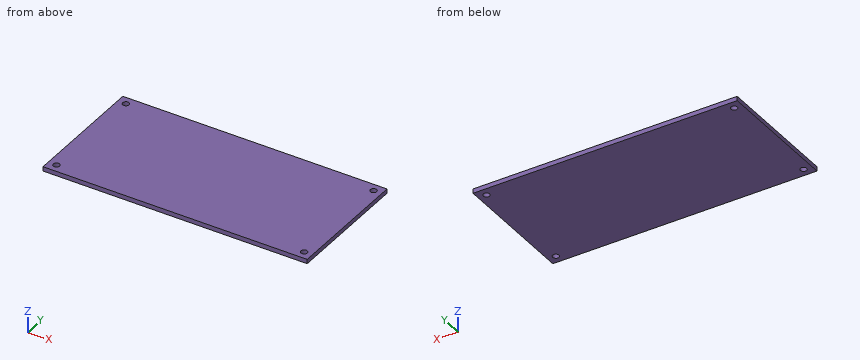
from build123d import *

# Parameters (mm, degrees)
ESQUISSE1_W        = 96
ESQUISSE1_H        = 46
ESQUISSE1_R        = 1.15
BOSS_EXTRU_1_DEPTH = 1.6


with BuildPart() as part:
    # Esquisse1 → Boss.-Extru.1 (new body)
    with BuildSketch(Plane.XY):
        Rectangle(ESQUISSE1_W, ESQUISSE1_H)
        with Locations((-45, 20)):
            Circle(ESQUISSE1_R, mode=Mode.SUBTRACT)
        with Locations(Location((45, 20, 0), (0, 0, 180))):
            Circle(ESQUISSE1_R, mode=Mode.SUBTRACT)
        with Locations(Location((-45, -20, 0), (0, 0, 180))):
            Circle(ESQUISSE1_R, mode=Mode.SUBTRACT)
        with Locations((45, -20)):
            Circle(ESQUISSE1_R, mode=Mode.SUBTRACT)
    extrude(amount=BOSS_EXTRU_1_DEPTH)


solid = part.part
Work out the finished part from the listing and answer in its coordinate system (mm). Give positions to 0.01 mm unless a question says otherwise; leave off trailing zeros. Write each loop counter-clockwise with the first axis right and the second up, starting at its lowest first coordinate (ties: lowest second). Pieces come first, ordered by that corner, then holes. Notation, with made-up numbers: (-9.5, 4) - (-4.5, 4) arc R27 ccw to (-4.5, 21) - close; hole circle Ø4 at (-36, -1.5). An arc over 180 degrees is marked (long way). One line per item, written item: value. Start each with the question number.
1. Given pin 1 (10 mm diameter, centred on x = -15.5, y = 3.5, fed in from -Z), flat-ended and moving along its own axis, determine where the tip first touches the part or whether it passes through.
2. Find section B-B (x = 45). Write down the section's boundary in (y, z).
3. Find section A-A (y = -20). Write down the section's boundary in (x, z), then the cut area to 3 significant figures.
4. Consider probe 1 along Y at (x, z) = (-45, 1.25); probe 2 along X at (y, z) = (19, 0.65). Determine where each line is inside the solid, lowest interval first.
Geometry results:
1. pin 1: z = 0
2. outline: (-23, 0) - (-21.15, 0) - (-21.15, 1.6) - (-23, 1.6) - close; (-18.85, 0) - (18.85, 0) - (18.85, 1.6) - (-18.85, 1.6) - close; (21.15, 0) - (23, 0) - (23, 1.6) - (21.15, 1.6) - close
3. outline: (-48, 0) - (-46.15, 0) - (-46.15, 1.6) - (-48, 1.6) - close; (-43.85, 0) - (43.85, 0) - (43.85, 1.6) - (-43.85, 1.6) - close; (46.15, 0) - (48, 0) - (48, 1.6) - (46.15, 1.6) - close
3. area: 146 mm2
4. probe 1: -23 to -21.15, -18.85 to 18.85, 21.15 to 23
4. probe 2: -48 to -45.57, -44.43 to 44.43, 45.57 to 48
